Check sheet for the modelled part. Datum: model origin and axes. Units: mm. A direction names the side the tool comes from. Coordinates: 2 decimals unless noted, no trailing zeros. Write each loop counter-clockwise with the first axis right and the second up, starting at its lowest first coordinate (ties: lowest second). Pieces come first, ordered by that corner, then holes. Notation, with made-up numbers: M 68,-18 L 115,-18 A22 cw 115,5 Z; hole C -13,5 d2. An arc over 180 degrees is marked long. Answer as CSV lines item,"result". Start each with the question number.
Q1. Sectioned sample at D-D, the plane x = 7. Record the cut outline in (y, z), then the cut area to 3 significant figures.
Q2. Sectioned sample at C-C, the plane y = 8.5. Record the cut outline in (x, z).
Q3. Access from +Z, -Z, +X, -X, +Y, -Y to the whole of each face (thin tool, end or side, straight path). Record for faces 4 (the flat face through (17, 6, 1)), 5 (the flat face through (9, 6.7, 9)), 6 (the flat face through (9, 9, 15)).
Q4. Depth check by flat-ended pin: pin 1 Ø3.5 at (x, z) = (5.5, 10) entering from -Y; pin 2 Ø2 at (x, y) = (11.5, 5) entering from +Z; pin 3 Ø4 at (x, z) = (12, 1) entering from -Y; pin 4 Ø3 at (y, z) = (7.5, 1) entering from +X. Enter the tip coordinate at first touch or a pass-through.
Q5. Sectioned sample at B-B, the plane z = 7.5. Record the cut outline in (x, y).
Q6. Sectioned sample at A-A, the plane y = 5.25. Record the cut outline in (x, z), then the cut area to 3 significant figures.
Q7. Mould release check, pull along X, two halves, no side actions. Record for faces 1 (the flat face through (9, 7.5, 2)), 2 (the flat face through (1, 0, 7)), 3 (the flat face through (0.8, 6, 1)): pulls with the +X half, pulls with the -X half, needs draft (parallel to the pull), parting line crosses it, or undercut.
Q8. Thickness scan on line 1 along X through (y, z) = (1.75, 12); line 2 along Y through (x, z) = (6.25, 8.5); line 3 along Y through (x, z) = (10.25, 2.25). Record the ranges inside material, lowest first. Write a range as from..to.
from build123d import *

# Parameters (mm, degrees)
SKETCH1_W           = 17.8
SKETCH1_H           = 12
BOSS_EXTRUDE1_DEPTH = 15
SKETCH2_W           = 14.8
SKETCH2_H           = 7.5
CUT_EXTRUDE1_DEPTH  = 27.188547115
SKETCH3_W           = 14.8
SKETCH3_H           = 11.449984897
BOSS_EXTRUDE2_DEPTH = 0.8
SKETCH4_W           = 0.8
SKETCH4_H           = 12
CUT_EXTRUDE2_DEPTH  = 2.7


with BuildPart() as part:
    # Sketch1 → Boss-Extrude1 (new body)
    with BuildSketch(Plane.XY):
        with Locations((8.9, 6)):
            Rectangle(SKETCH1_W, SKETCH1_H)
    extrude(amount=BOSS_EXTRUDE1_DEPTH)

    # Sketch2 → Cut-Extrude1 (cut, through all)
    with BuildSketch(Plane.XY.offset(15)):
        with Locations((8.9, 3.75)):
            Rectangle(SKETCH2_W, SKETCH2_H)
    extrude(amount=-CUT_EXTRUDE1_DEPTH, mode=Mode.SUBTRACT)

    # Sketch3 → Boss-Extrude2 (add)
    with BuildSketch(Plane.XZ.offset(-7.5)):
        with Locations((8.9, 9.275007552)):
            Rectangle(SKETCH3_W, SKETCH3_H)
    extrude(amount=BOSS_EXTRUDE2_DEPTH)

    # Sketch4 → Cut-Extrude2 (cut)
    with BuildSketch(Plane(origin=(0, 0, 0), x_dir=(-1, 0, 0), z_dir=(0, 0, -1))):
        with Locations((-17.4, 6)):
            Rectangle(SKETCH4_W, SKETCH4_H)
        with Locations((-0.4, 6)):
            Rectangle(SKETCH4_W, SKETCH4_H)
    extrude(amount=-CUT_EXTRUDE2_DEPTH, mode=Mode.SUBTRACT)


solid = part.part
Output:
1,outline,"M 6.7,3.55 L 7.5,3.55 L 7.5,0 L 12,0 L 12,15 L 6.7,15 Z"
1,area,"76.7 mm^2"
2,outline,"M 0,2.7 L 0.8,2.7 L 0.8,0 L 17,0 L 17,2.7 L 17.8,2.7 L 17.8,15 L 0,15 Z"
3,face 4,"-Z, +X, +Y, -Y"
3,face 5,"+Z, -Z, -Y"
3,face 6,"+Z, +X, -X, +Y, -Y"
4,pin 1,"stops at y = 6.7"
4,pin 2,"passes through"
4,pin 3,"stops at y = 7.5"
4,pin 4,"stops at x = 17"
5,outline,"M 0,0 L 1.5,0 L 1.5,6.7 L 16.3,6.7 L 16.3,0 L 17.8,0 L 17.8,12 L 0,12 Z"
6,outline,"M 0,2.7 L 0.8,2.7 L 0.8,0 L 1.5,0 L 1.5,15 L 0,15 Z; M 16.3,0 L 17,0 L 17,2.7 L 17.8,2.7 L 17.8,15 L 16.3,15 Z"
6,area,"40.7 mm^2"
7,face 1,"undercut"
7,face 2,"needs draft"
7,face 3,"pulls with the -X half"
8,line 1,"x = 0..1.5, 16.3..17.8"
8,line 2,"y = 6.7..12"
8,line 3,"y = 7.5..12"
